Check sheet for the drawn part. Datum: minimum x, y, z corner. Units: mm. Round coordinates to 2 decimals unless told otherwise and drop trailing zeros. Order: outer loops, then holes, each group sorted by start corner. A loop starts at its lowest first (then second) coordinate and runs counter-clockwise, first axis right, second up. Notation, with made-up numbers: (34.25, 2.25) -> (92.25, 2.25) arc R20 cw to (92.25, 23.25) -> close; hole circle Ø5 at (-26.5, -33.75). An arc over 180 degrees is marked (long way). Answer as a JSON object with one key per item and string values. Group by question number.
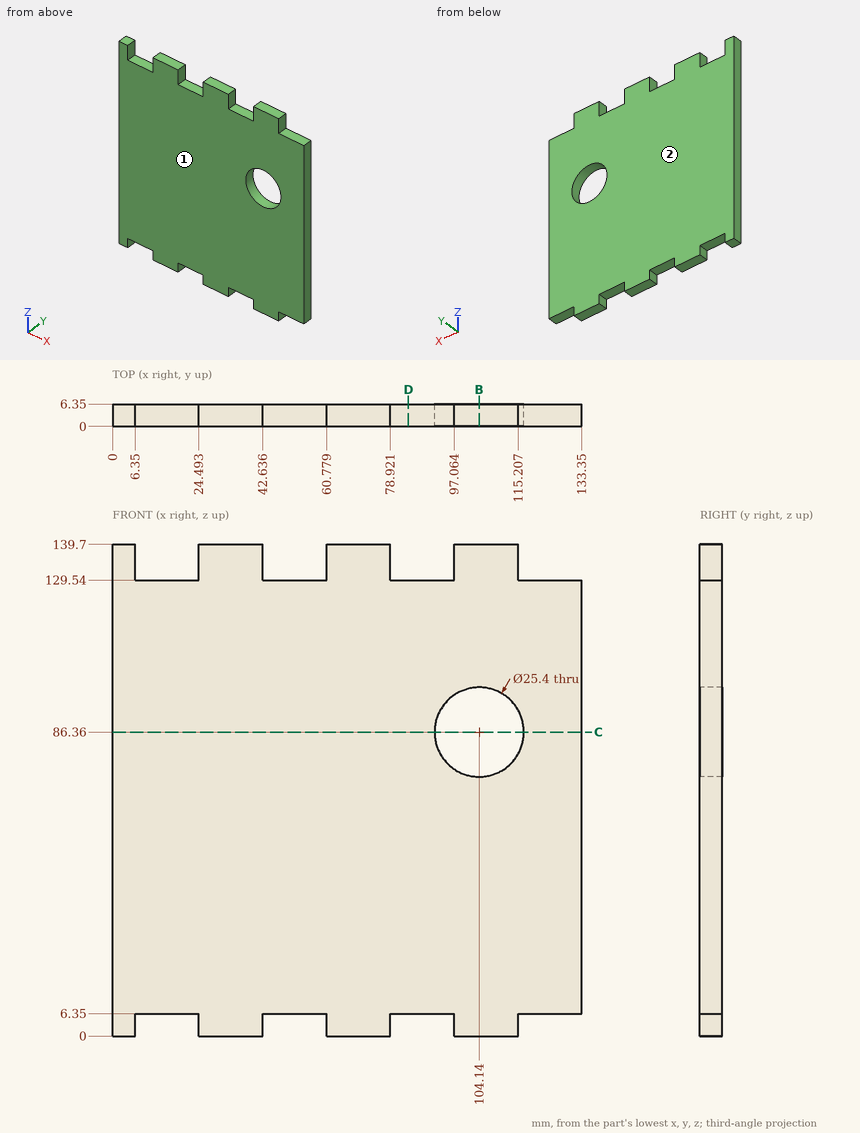
Item 1: Sectioned sample at C-C, the plane z = 86.36. Enter the section's corners in (x, y).
Item 2: Depth check by flat-ended pin: pin 1 Ø3 at (y, z) = (3.5, 4.5) entering from +X; pin 2 Ø3 at (y, z) = (3.5, 135) entering from -X; pin 3 Ø1.9 at (x, y) = (85.5, 2) entering from -Z. Enter the tip coordinate at first touch or a pass-through.
Item 3: Thickness scan on L1, parallel to Z at x = 104.14, y = 4.75; L2, parallel to Z at x = 51.5, y = 2.5; L3, parallel to Z at x = 114.5, y = 4.75 (1 decimal). Record the ranges inside material, lowest first.
Item 4: Sectioned sample at D-D, the plane x = 84. Enter the section's corners in (y, z), then the cut area to 3 significant figures.
Item 5: Sectioned sample at B-B, the plane x = 104.14. Enter the section's corners in (y, z), then the cut area to 3 significant figures.
Item 6: Mould release check, pull along Y, two halves, no side actions. Record for the marked faces 1 and 2: pulls with the +Y half, pulls with the -Y half, needs draft (parallel to the pull), parting line crosses it, or undercut.
Result:
{
 "1": {"outline": "(0, 0) -> (91.44, 0) -> (91.44, 6.35) -> (0, 6.35) -> close; (116.84, 0) -> (133.35, 0) -> (133.35, 6.35) -> (116.84, 6.35) -> close"},
 "2": {"pin 1": "stops at x = 115.21", "pin 2": "stops at x = 0", "pin 3": "stops at z = 6.35"},
 "3": {"L1": "z = 0 to 73.66, 99.06 to 139.7", "L2": "z = 6.35 to 129.54", "L3": "z = 0 to 79, 93.7 to 139.7"},
 "4": {"outline": "(0, 6.35) -> (6.35, 6.35) -> (6.35, 129.54) -> (0, 129.54) -> close", "area": "782 mm2"},
 "5": {"outline": "(0, 0) -> (6.35, 0) -> (6.35, 73.66) -> (0, 73.66) -> close; (0, 99.06) -> (6.35, 99.06) -> (6.35, 139.7) -> (0, 139.7) -> close", "area": "726 mm2"},
 "6": {"face 1": "pulls with the -Y half", "face 2": "pulls with the +Y half"}
}
